Source: CAD feature listing. Evaluate the final solid. Frame: model axes, mm. Coordinates: 2 decimals unless noted, no trailing zeros. Order: outer loops, then holes, each group sorted by start corner. A loop starts at its lowest first (then second) coordinate and runs counter-clockwise, first axis right, second up. Notation, with made-up numbers: (-17.75, 69.5) - (24.25, 69.5) arc R25 cw to (24.25, 105.5) - close; hole circle Ø11 at (59.5, 1.25). An arc over 180 degrees is marked (long way). One line per question, with ' | ' between items.
Autodesk Inventor part; units mm, degrees
ref_plane "YZ Plane" through (0, 0, 0) normal (1, 0, 0) x (0, 1, 0)
ref_plane "XZ Plane" through (0, 0, 0) normal (0, 1, 0) x (-1, 0, 0)
ref_plane "XY Plane" through (0, 0, 0) normal (0, 0, 1) x (1, 0, 0)
sketch "Sketch1" plane through (0, 0, 0) normal (0, 1, 0) x (-1, 0, 0)
  line L0 (6.35, 15.875) -> (-6.35, 15.875)
  line L1 (-6.35, 15.875) -> (-6.35, -15.875)
  line L2 (-6.35, -15.875) -> (6.35, -15.875)
  line L3 (6.35, -15.875) -> (6.35, 15.875)
  line L4 (6.35, 15.875) -> (-6.35, -15.875) construction
  line L5 (-6.35, 15.875) -> (6.35, -15.875) construction
  point P0 (0, 0)
  dimension "d0" = 31.75
  dimension "d1" = 12.7
extrude "Plate1" add sketch "Sketch1" along normal blind 12.7
sketch "Sketch2" plane through (6.35, 0, 15.875) normal (1, 0, 0) x (0, 0, -1)
  line L0 (0, 0) -> (0, 12.7) construction
  point P0 (15.875, 0)
  point P1 (6.35, 6.35)
  point P2 (19.05, 6.35)
  point P3 (0, 6.35)
  dimension "d3" = 12.7
  dimension "d4" = 6.35
hole "Hole1" at (6.35, 6.35, 9.525) at (6.35, 6.35, -3.175) direction (-1, 0, 0) diameter 3.9624 end through all
sketch "Sketch3" plane through (0, 12.7, 0) normal (0, 1, 0) x (1, 0, 0)
  point P0 (0, 0)
  point P1 (0, -3.175)
  point P2 (0, 9.525)
  dimension "d12" = 12.7
  dimension "d13" = 3.175
hole "Hole2" at (0, 12.7, 3.175) at (0, 12.7, -9.525) direction (0, -1, 0) diameter 3.9624 end through all
fillet "Corner Round1" radius 1.5875 4 edges at (6.35, 6.35, 15.875) (-6.35, 6.35, 15.875) (-6.35, 6.35, -15.875) (6.35, 6.35, -15.875)
equation "\"d2\" = Thickness"
equation "\"BendRadius\" = Thickness"
equation "\"BendReliefWidth\" = Thickness"
equation "\"BendReliefDepth\" = 0.5 * Thickness"
equation "\"CornerReliefSize\" = 4 * Thickness"
equation "\"MinimumRemnant\" = 2 * Thickness"
equation "\"TransitionRadius\" = BendRadius"
equation "\"JacobiRadiusSize\" = BendRadius"
equation "\"GapSize\" = Thickness"
properties part number "PLATE,NUTBLOCK" material "Aluminum 6061"
(1) Cut plane D-D (z = -9.5). Return the cut outline in (x, y).
Taken from the geometry:
outline: (-6.35, 0) - (-1.98, 0) - (-1.98, 12.7) - (-6.35, 12.7) - close; (1.98, 0) - (6.35, 0) - (6.35, 12.7) - (1.98, 12.7) - close
(2) Pin query (flat end, axial travel): P1, Ø2.5, axis at x = 0, z = -9.525, coming from the -Y side. Return the tip coordinate at first contact, or that it passes through.
Taken from the geometry:
P1: passes through
(3) Cut plane B-B (x = 0). Return the cut outline in (y, z) (3 decimals).
Taken from the geometry:
outline: (0, -15.875) - (12.7, -15.875) - (12.7, -11.506) - (0, -11.506) - close; (0, -7.544) - (12.7, -7.544) - (12.7, 1.194) - (0, 1.194) - close; (0, 5.156) - (12.7, 5.156) - (12.7, 15.875) - (0, 15.875) - close; hole circle Ø3.962 at (6.35, -3.175); hole circle Ø3.962 at (6.35, 9.525)
(4) Cut plane A-A (y = 6.35). State how many separate pieces and enclosed holes the cut face has, and give its area (3 significant figures).
Taken from the geometry:
separate pieces: 3 | enclosed holes: 2 | area: 276 mm²
(5) Material intervals for L1, parallel to Z at x = -4, y = 6.25 (3 decimals); L2, parallel to Z at x = 0.5, y = 6.35 (3 decimals); L3, parallel to Z at x = 0, y = 3.75 (3 decimals), sorted ascending. Write a range as from..to.
Taken from the geometry:
L1: z = -15.875..-5.154, -1.196..7.546, 11.504..15.875 | L2: z = -15.875..-11.442, -7.608..-5.156, -1.194..1.258, 5.092..7.544, 11.506..15.875 | L3: z = -15.875..-11.506, -7.544..1.194, 5.156..15.875
(6) Pull-direction query (Z, two-part tool) for faces 1 (the cylindrical face through (5.897, 6.439, -15.398)), 2 (the flat face through (6.35, 6, 0)), 3 (the cylindrical face through (-1.339, 6.261, 1.715)); classes: pulls with the +Z half, pulls with the -Z half, needs draft (parallel to the pull), parting line crosses it, or undercut.
Taken from the geometry:
face 1: pulls with the -Z half | face 2: needs draft | face 3: undercut
